Read the model definition and answer for the solid it produces. Units are mm, in the model's axes. Face numbers are marked on the shaded views. A direction names the side the tool comes from. Round coordinates to 2 decimals unless told otherwise and drop trailing zeros. Order: outer loops, then holes, each group sorted by start corner. A loop starts at its lowest first (then second) coordinate and runs counter-clockwise, first axis right, second up. Notation, with made-up numbers: (54.5, 67) -> (74.5, 67) arc R25 cw to (74.5, 102) -> close; hole circle Ø8 at (-9.75, 67). An arc over 180 degrees is marked (long way). Answer as a JSON object with one key per item and string values. Group by question number.
Item 1: Given P1, Ø16, axis at y = 43, z = 29, coming from the +X side; P2, Ø8, axis at x = 32.5, y = 40.5, coming from the +Z side; P3, Ø12, axis at y = 53, z = 6.5, coming from the -X side, each flat-ended and moving along its own axis, determine where each tip first touches the part or whether it passes through.
Item 2: For the marked faces 1, 2 and 3, determine the directions among +Z, -Z, +X, -X, +Y, -Y from which every point of the face is accessible in a straight line to the end or side of a thin tool.
Item 3: The mould has two halves that part along X. Classify the marked faces 4, 5 and 6: pulls with the +X half, pulls with the -X half, needs draft (parallel to the pull), parting line crosses it, or undercut.
Item 4: Section C-C, the plane x = 0 is taken. Write down the section's boundary in (y, z), plus the area to 3 significant figures.
Item 5: Section D-D, the plane z = -19 is taken. Write down the section's boundary in (x, y).
Item 6: Consider probe 1 along X at (y, z) = (22, 27); probe 2 along X at (y, z) = (61, 0.5); probe 3 along Z at (x, y) = (-5, 28). Determine where each line is inside the solid, lowest interval first. Write a range as from..to.
Item 7: Section B-B, the plane y = 67 is taken. Write down the section's boundary in (x, z), plus the area to 3 significant figures.
Item 8: Section A-A, the plane z = 0.5 is taken. Write down the section's boundary in (x, y).
Solid Edge part; units mm, degrees
sketch "Sketch1" plane through (0, 0, 0) normal (0, -1, 0) x (1, 0, 0)
  circle A0 centre (0, 0) radius 35
extrude "Protrusion1" add sketch "Sketch1" against normal blind 90
sketch "Sketch2" plane through (0, 0, 0) normal (0, -1, 0) x (1, 0, 0)
  line L0 (-4, 35) -> (-4, 20)
  line L1 (-4, 35) -> (4, 35)
  line L2 (4, 20) -> (4, 35)
  arc A0 (4, 20) -> (-4, 20) centre (0, 20) cw
extrude "ExtrudedCutout_1" cut sketch "Sketch2" against normal blind 90 and the other way blind 1
sketch "Sketch3" plane through (0, 0, -0.1147) normal (0, -1, 0) x (0, 0, -1)
  line L0 (6.8853, 34.2929) -> (6.8853, 27)
  line L1 (6.8853, 27) -> (22.1564, 27)
  arc A0 (22.1564, 27) -> (6.8853, 34.2929) centre (-0.1147, 0) ccw
  line L2 (-7.1147, 34.2929) -> (-7.1147, 27)
  line L3 (-7.1147, 27) -> (-22.3857, 27)
  arc A1 (-22.3857, 27) -> (-7.1147, 34.2929) centre (-0.1147, 0) cw
extrude "ExtrudedCutout_2" cut sketch "Sketch3" against normal blind 90 and the other way blind 1
sketch "Sketch4" plane through (0, 0, -0.1147) normal (0, -1, 0) x (1, 0, 0)
  line L0 (17.5402, -34.8853) -> (-17.5, -34.8853)
  line L1 (-17.5, -34.8853) -> (-8.7575, 2.1803)
  line L2 (17.5402, -34.8853) -> (8.7554, 2.1892)
  arc A0 (-8.7575, 2.1803) -> (8.7554, 2.1892) centre (0, 0.1147) cw
extrude "ExtrudedCutout_3" cut sketch "Sketch4" against normal blind 90 and the other way blind 1
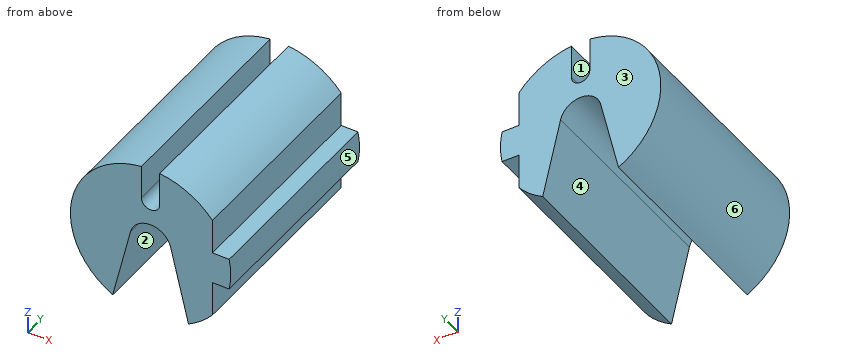
Values found:
{
 "1": {"P1": "x = 27", "P2": "z = 7", "P3": "x = -35"},
 "2": {"face 1": "+Z, +Y, -Y", "face 2": "-Z, +Y, -Y", "face 3": "+Z, -Z, +X, -X, +Y"},
 "3": {"face 4": "undercut", "face 5": "pulls with the +X half", "face 6": "pulls with the -X half"},
 "4": {"outline": "(0, 9) -> (90, 9) -> (90, 16) -> (0, 16) -> close", "area": "630 mm2"},
 "5": {"outline": "(-29.39, 0) -> (-13.73, 0) -> (-13.73, 90) -> (-29.39, 90) -> close; (13.75, 0) -> (27, 0) -> (27, 90) -> (13.75, 90) -> close"},
 "6": {"probe 1": "-22.27..-4, 4..22.27", "probe 2": "-35..-9.13, 9.13..35", "probe 3": "7.48..34.64"},
 "7": {"outline": "(-16.52, -30.85) -> (-8.76, 2.07) arc R9 cw to (8.76, 2.07) -> (16.55, -30.84) arc R35 ccw to (27, -22.27) -> (27, -7) -> (34.29, -7) arc R35 ccw to (34.29, 7) -> (27, 7) -> (27, 22.27) arc R35 ccw to (4, 34.77) -> (4, 20) arc R4 cw to (-4, 20) -> (-4, 34.77) arc R35 ccw to start", "area": "2,550 mm2"},
 "8": {"outline": "(-35, 0) -> (-9.13, 0) -> (-9.13, 90) -> (-35, 90) -> close; (9.13, 0) -> (35, 0) -> (35, 90) -> (9.13, 90) -> close"}
}
